from build123d import *

# Parameters (mm, degrees)
F1_DEPTH = 122
F3_DEPTH = 11
F5_DEPTH = 8.001


with BuildPart() as f1:
    # F0 (on Front) → F1 (new body)
    with BuildSketch(Plane.XZ):
        with BuildLine():
            Line((-13, 5.003651), (-69, 5.003651))
            Line((-69, 5.003651), (-69, -2.996349))
            Line((-69, -2.996349), (0.385778, -2.996349))
            add(Edge.make_bspline(
                [(-13, 5.003651), (-8, 5.003651), (-4.435703, 1.439354), (-0.871407, -2.124942), (0.385778, -2.996349)],
                knots=[0, 0, 0, 0, 11.18034, 15.940018, 15.940018, 15.940018, 15.940018], degree=3))
        make_face()
    extrude(amount=F1_DEPTH)

    # F2 (on face) → F3 (join)
    with BuildSketch(Plane.XY.offset(5.003651)):
        with BuildLine():
            ThreePointArc((-69, -84.18975), (-57.958933, -67.473303), (-39, -61))
            ThreePointArc((-39, -61), (-57.958933, -54.526697), (-69, -37.81025))
            Line((-69, -37.81025), (-69, -84.18975))
        make_face()
    extrude(amount=F3_DEPTH)

    # F4 (on face) → F5 (cut, through all)
    with BuildSketch(Plane.XY.offset(5.003651)):
        with BuildLine():
            ThreePointArc((-39, -122), (-60.213203, -113.213203), (-69, -92))
            Line((-69, -92), (-69, -122))
            Line((-69, -122), (-39, -122))
        make_face()
        with BuildLine():
            Line((-69, 0), (-69, -30))
            ThreePointArc((-69, -30), (-60.213203, -8.786797), (-39, 0))
            Line((-39, 0), (-69, 0))
        make_face()
    extrude(amount=-F5_DEPTH, mode=Mode.SUBTRACT)


solid = f1.part
Verification items for the finished model (mm, model axes). A direction names the side the tool comes from. Round coordinates to 2 decimals unless told otherwise and drop trailing zeros. Loops run counter-clockwise (first coordinate to the right, second up) from the corner with the lowest first, then second, coordinate; pieces in that order, holes last. Notation, with made-up numbers: (77.5, 46.5) - (115.5, 46.5) arc R33 cw to (115.5, 77.5) - close; hole circle Ø11 at (40.5, 6). An arc over 180 degrees is marked (long way). Write item = value, one per line.
Q1. Sectioned sample at C-C on x = -60.5. Record the boundary of the cut face in (y, z).
Here are the results:
outline = (-112.92, -3) - (-9.08, -3) - (-9.08, 5) - (-52.33, 5) - (-52.33, 16) - (-69.67, 16) - (-69.67, 5) - (-112.92, 5) - close
Q2. Tool access check on faces 1 (the flat face through (-41, -60, 5.004)), 2 (the cylindrical face through (-58.184, -67.649, 10.427)), 3 (the cylindrical face through (-57.73, -54.7, 10.43)), 4 (the flat face through (-69, -61, 7)). Record the directions out of +Z, -Z, +X, -X, +Y, -Y that give a thin tool (end or side, any length) a straight path to the whole face; none if there is none.
Here are the results:
face_1 = +Z, +X
face_2 = +Z, +X, -Y
face_3 = +Z, +X, +Y
face_4 = +Z, -Z, -X, +Y, -Y
Q3. Sectioned sample at B-B on z = 10. Record the boundary of the cut face in (x, y), plus the area to 3 significant figures.
Here are the results:
outline = (-69, -84.19) arc R31 cw to (-39, -61) arc R31 cw to (-69, -37.81) - close
area = 361 mm^2
Q4. Depth check by flat-ended pin: pin 1 (17 mm diameter, centred on x = -43.5, y = -35.5, fed in from +Z); pin 2 (1 mm diameter, centred on x = -53.5, z = 7.5, fed in from +Y); pin 3 (6 mm diameter, centred on x = -45.5, z = 1, fed in from -Y). Enter the tip coordinate at first touch or a pass-through.
Here are the results:
pin_1 = 5
pin_2 = -57.13
pin_3 = -121.8
Q5. Material ranges on L1, parallel to Z at x = -44, y = -20; L2, parallel to Y at x = -51.5, z = 8.5; L3, parallel to X at y = -38.5, z = 9.25, recorded low to high.
Here are the results:
L1 = -3 to 5
L2 = -63.63 to -58.37
L3 = -69 to -68.81
Q6. Sectioned sample at A-A on x = -33. Record the boundary of the cut face in (y, z).
Here are the results:
outline = (-122, -3) - (0, -3) - (0, 5) - (-122, 5) - close
